The listing builds one solid part. Answer for the finished solid, in the listing's coordinates (mm). Face numbers are marked on the shaded views. A direction names the side the tool comes from. Give positions to 0.01 mm unless a question says otherwise; leave off trailing zeros. Loops run counter-clockwise (first coordinate to the right, second up) from the corner with the lowest first, then second, coordinate; pieces in that order, holes last. Notation, with made-up numbers: (46, 54) - (95, 54) arc R20 ccw to (95, 74) - close; hole circle Ø7 at (62.25, 44.25). An arc over 180 degrees is marked (long way). One line per item, written item: value. Start each with the question number.
from build123d import *

# Parameters (mm, degrees)
SKETCH1_R                    = 8.89
BOSS_EXTRUDE2_DEPTH          = 19.05
SHELL7_T                     = -2.54
SKETCH3_R                    = 8.89
BOSS_EXTRUDE4_DEPTH          = 3.175
SKETCH4_W                    = 50.8
SKETCH4_H                    = 17.006105847
BOSS_EXTRUDE5_DEPTH          = 3.175
SKETCH5_W                    = 3.81
SKETCH5_H                    = 3.15
CUT_REVOLVE1_ANGLE           = 60
CUT_REVOLVE1_OTHER_WAY_ANGLE = 60
SKETCH6_R                    = 0.762
CUT_EXTRUDE1_DEPTH           = 39.937338239
CUT_EXTRUDE1_DEPTH_BACK      = 39.937338239
CUT_EXTRUDE2_DEPTH           = 36.565821813


with BuildPart() as part:
    # Sketch1 → Boss-Extrude2 (new body)
    with BuildSketch(Plane(origin=(0, 0, 0), x_dir=(1, 0, 0), z_dir=(0, 1, 0))):
        with Locations(Location((0, 0, 0), (0, 0, 90))):
            Circle(SKETCH1_R)
    extrude(amount=BOSS_EXTRUDE2_DEPTH)

    # Shell7
    shell7_openings = [part.faces().sort_by_distance(p)[0] for p in [
        (0, 0, 0),
    ]]
    offset(amount=SHELL7_T, openings=shell7_openings, kind=Kind.INTERSECTION)

    # Sketch3 → Boss-Extrude4 (add)
    with BuildSketch(Plane(origin=(0, 19.05, 0), x_dir=(1, 0, 0), z_dir=(0, 1, 0))):
        with Locations(Location((0, 0, 0), (0, 0, 90))):
            Circle(SKETCH3_R)
    extrude(amount=BOSS_EXTRUDE4_DEPTH)

    # Sketch4 → Boss-Extrude5 (add)
    with BuildSketch(Plane(origin=(0, 22.225, 0), x_dir=(1, 0, 0), z_dir=(0, 1, 0))):
        with Locations((-0.90484663, -0.237125368)):
            Rectangle(SKETCH4_W, SKETCH4_H)
    extrude(amount=BOSS_EXTRUDE5_DEPTH)

    # Sketch5 → Cut-Revolve1 (revolve, cut)
    with BuildSketch(Plane(origin=(0, 0, -0.018592303), x_dir=(-1, 0, 0), z_dir=(0, 0, -1))):
        with Locations((-6.985, 8.255)):
            Rectangle(SKETCH5_W, SKETCH5_H)
        with Locations((6.985, 8.255)):
            Rectangle(SKETCH5_W, SKETCH5_H)
    revolve(axis=Axis((0, 0, -0.018592303), (0, 1, 0)), revolution_arc=CUT_REVOLVE1_ANGLE, mode=Mode.SUBTRACT)

    # Sketch5 → Cut-Revolve1 other way (revolve, cut)
    with BuildSketch(Plane(origin=(0, 0, -0.018592303), x_dir=(-1, 0, 0), z_dir=(0, 0, -1))):
        with Locations((-6.985, 8.255)):
            Rectangle(SKETCH5_W, SKETCH5_H)
        with Locations((6.985, 8.255)):
            Rectangle(SKETCH5_W, SKETCH5_H)
    revolve(axis=Axis((0, 0, -0.018592303), (0, -1, 0)), revolution_arc=CUT_REVOLVE1_OTHER_WAY_ANGLE, mode=Mode.SUBTRACT)

    # Sketch6 → Cut-Extrude1 (cut, two sides)
    with BuildSketch(Plane(origin=(0, 0, -4.489512434), x_dir=(-1, 0, 0), z_dir=(0, 0, -1))) as cut_extrude1_sk:
        with Locations((-11.839923773, 23.8125)):
            Circle(SKETCH6_R)
        with Locations((11.839923773, 23.8125)):
            Circle(SKETCH6_R)
    extrude(amount=CUT_EXTRUDE1_DEPTH, mode=Mode.SUBTRACT)
    extrude(cut_extrude1_sk.sketch, amount=-CUT_EXTRUDE1_DEPTH_BACK, mode=Mode.SUBTRACT)

    # Sketch7 → Cut-Extrude2 (cut, through all)
    with BuildSketch(Plane(origin=(0, 22.225, 0), x_dir=(1, 0, 0), z_dir=(0, 1, 0))):
        with BuildLine():
            Line((-3.272085213, 8.265927556), (3.272085213, 8.265927556))
            ThreePointArc((3.272085213, 8.265927556), (0, 8.89), (-3.272085213, 8.265927556))
        make_face()
    extrude(amount=-CUT_EXTRUDE2_DEPTH, mode=Mode.SUBTRACT)


solid = part.part
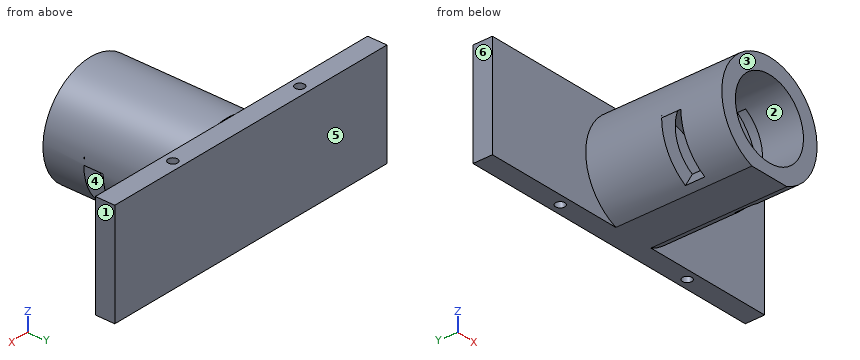
1. Flat-ended cylindrical pins translate along their axes: pin 1 (7.5 mm diameter, centred on x = 0, z = 0, fed in from -Y); pin 2 (8.5 mm diameter, centred on x = 16, z = 3.5, fed in from -Y) (3 decimals); pin 3 (1 mm diameter, centred on x = 3, y = 9.5, fed in from +Z). Find the tip coordinate at first contact, or state that the pin passes through.
2. A cutting plane is placed at C-C (z = 2.5). Determine the outline of the cut face in (x, y) (1 decimal), plus the area to 3 significant figures.
3. A cutting plane is placed at D-D (x = 0). Determine the outline of the cut face in (y, z) (3 decimals), plus the area to 3 significant figures.
4. A cutting plane is placed at A-A (z = -4). Determine the outline of the cut face in (x, y) (1 decimal), plus the area to 3 significant figures.
5. Find the intervals of material crossed by L1, parallel to X at y = 11.5, z = 0; L2, parallel to X at y = 23.25, z = -5.5; L3, parallel to Z at x = 15, y = 23.25, in increasing order. Write a range as [from, to].
6. A cutting plane is placed at B-B (y = 8.5). Determine the outline of the cut face in (x, z) (3 decimals), plus the area to 3 significant figures.
7. For the marked faces 1 and 2, determine the directions among +Z, -Z, +X, -X, +Y, -Y from which every point of the face is accessible in a straight line to the end or side of a thin tool.
8. Determine the mould class of the marked faces 3, 4, 5 and 6 for opening direction Y: released by +Y, released by -Y, zero draft, split by the parting line, or undercut.
Results below:
1. pin 1: stops at y = 16.51
1. pin 2: stops at y = 22.225
1. pin 3: stops at z = 8.53
2. outline: (-26.3, 22.2) - (-8.5, 22.2) - (-8.5, 0) - (-5.8, 0) - (-5.8, 6.7) - (-8.5, 6.7) - (-8.5, 9.8) - (-5.8, 9.8) - (-5.8, 16.5) - (5.8, 16.5) - (5.8, 9.8) - (8.5, 9.8) - (8.5, 6.7) - (5.8, 6.7) - (5.8, 0) - (8.5, 0) - (8.5, 22.2) - (24.5, 22.2) - (24.5, 25.4) - (-26.3, 25.4) - close; hole circle Ø1.5 at (-11.8, 23.8); hole circle Ø1.5 at (11.8, 23.8)
2. area: 327 mm^2
3. outline: (0, -8.266) - (25.4, -8.266) - (25.4, 8.74) - (22.225, 8.74) - (22.225, 8.89) - (0, 8.89) - (0, 6.35) - (16.51, 6.35) - (16.51, -6.35) - (0, -6.35) - close
3. area: 226 mm^2
4. outline: (-26.3, 22.2) - (-7.9, 22.2) - (-7.9, 9.8) - (-4.9, 9.8) - (-4.9, 16.5) - (4.9, 16.5) - (4.9, 9.8) - (7.9, 9.8) - (7.9, 22.2) - (24.5, 22.2) - (24.5, 25.4) - (-26.3, 25.4) - close; (-7.9, 0) - (-4.9, 0) - (-4.9, 6.7) - (-7.9, 6.7) - close; (4.9, 0) - (7.9, 0) - (7.9, 6.7) - (4.9, 6.7) - close; hole circle Ø1.5 at (-11.8, 23.8); hole circle Ø1.5 at (11.8, 23.8)
4. area: 329 mm^2
5. L1: x = [-8.89, -6.35], [6.35, 8.89]
5. L2: x = [-26.3, -12.35], [-11.33, 11.33], [12.35, 24.5]
5. L3: z = [-8.27, 8.74]
6. outline: (-8.89, -0.009) arc R8.89 cw to (-4.445, 7.68) - (-3.183, 5.495) arc R6.35 cw to (3.183, 5.495) - (4.445, 7.68) arc R8.89 cw to (8.89, -0.009) arc R8.89 ccw to start; (-4.437, -7.704) arc R8.89 ccw to (-3.272, -8.266) - (3.272, -8.266) arc R8.89 ccw to (4.437, -7.704) - (3.167, -5.504) arc R6.35 cw to (-3.167, -5.504) - close
6. area: 38.0 mm^2
7. face 1: +Z, -Z, +X, +Y, -Y
7. face 2: -Y
8. face 3: released by -Y
8. face 4: undercut
8. face 5: released by +Y
8. face 6: zero draft
